```python
from build123d import *

# Parameters (mm, degrees)
EXTRUDE1_DEPTH     = 50.8
CUT_EXTRUDE1_DEPTH = 9.525
SKETCH3_R          = 2.38125
CUT_EXTRUDE2_DEPTH = 15.875
CUT_EXTRUDE3_START = -15.875
SKETCH4_R          = 2.38125
CUT_EXTRUDE3_DEPTH = 15.875
CUT_EXTRUDE4_DEPTH = 222.795964766
EXTRUDE2_DEPTH     = 50.8


with BuildPart() as part:
    # Sketch1 → Extrude1 (new body)
    with BuildSketch(Plane.XY):
        Polygon((0, 0), (215.526146874, 0), (202.826146874, 12.7), (5.260512242, 12.7), align=None)
    extrude(amount=EXTRUDE1_DEPTH)

    # Sketch2 → Cut-Extrude1 (cut)
    with BuildSketch(Plane(origin=(0, 12.7, 0), x_dir=(-1, 0, 0), z_dir=(0, 1, 0))):
        with BuildLine():
            Line((-183.776146874, 41.275), (-116.743329558, 41.275))
            ThreePointArc((-116.743329558, 41.275), (-112.253201498, 39.415128061), (-110.393329558, 34.925))
            Line((-110.393329558, 34.925), (-110.393329558, 15.875))
            ThreePointArc((-110.393329558, 15.875), (-112.253201498, 11.384871939), (-116.743329558, 9.525))
            Line((-116.743329558, 9.525), (-183.776146874, 9.525))
            ThreePointArc((-183.776146874, 9.525), (-188.266274935, 11.384871939), (-190.126146874, 15.875))
            Line((-190.126146874, 15.875), (-190.126146874, 34.925))
            ThreePointArc((-190.126146874, 34.925), (-188.266274935, 39.415128061), (-183.776146874, 41.275))
        make_face()
        with BuildLine():
            Line((-91.343329558, 9.525), (-24.310512242, 9.525))
            ThreePointArc((-24.310512242, 9.525), (-19.820384182, 11.384871939), (-17.960512242, 15.875))
            Line((-17.960512242, 15.875), (-17.960512242, 34.925))
            ThreePointArc((-17.960512242, 34.925), (-19.820384182, 39.415128061), (-24.310512242, 41.275))
            Line((-24.310512242, 41.275), (-91.343329558, 41.275))
            ThreePointArc((-91.343329558, 41.275), (-95.833457619, 39.415128061), (-97.693329558, 34.925))
            Line((-97.693329558, 34.925), (-97.693329558, 15.875))
            ThreePointArc((-97.693329558, 15.875), (-95.833457619, 11.384871939), (-91.343329558, 9.525))
        make_face()
    extrude(amount=-CUT_EXTRUDE1_DEPTH, mode=Mode.SUBTRACT)

    # Sketch3 → Cut-Extrude2 (cut)
    with BuildSketch(Plane.XY.offset(50.8)):
        with Locations((101.226146874, 6.35)):
            Circle(SKETCH3_R)
    extrude(amount=-CUT_EXTRUDE2_DEPTH, mode=Mode.SUBTRACT)

    # Sketch4 → Cut-Extrude3 (cut)
    with BuildSketch(Plane(origin=(0, 0, 0), x_dir=(-1, 0, 0), z_dir=(0, 0, -1)).offset(CUT_EXTRUDE3_START)):
        with Locations(Location((-101.226146874, 6.35, 0), (0, 0, 180))):
            Circle(SKETCH4_R)
    extrude(amount=CUT_EXTRUDE3_DEPTH, mode=Mode.SUBTRACT)

    # Sketch5 → Cut-Extrude4 (cut, through all)
    with BuildSketch(Plane.XY.offset(50.8)):
        with BuildLine():
            Line((0.800865302, 1.933459874), (0, 0))
            Line((0, 0), (10.521024484, 0))
            ThreePointArc((10.521024484, 0), (5.565730305, 0.488053878), (0.800865302, 1.933459874))
        make_face()
    extrude(amount=-CUT_EXTRUDE4_DEPTH, mode=Mode.SUBTRACT)

    # Sketch6 → Extrude2 (add)
    with BuildSketch(Plane.XY.offset(50.8)):
        with BuildLine():
            Line((5.660944893, 13.666729937), (5.260512242, 12.7))
            Line((5.260512242, 12.7), (10.521024484, 12.7))
            ThreePointArc((10.521024484, 12.7), (8.043377395, 12.944026939), (5.660944893, 13.666729937))
        make_face()
    extrude(amount=-EXTRUDE2_DEPTH)


solid = part.part
```
Verification items for the finished model (mm, model axes). A direction names the side the tool comes from. Coordinates: 2 decimals unless noted, no trailing zeros. Loops run counter-clockwise (first coordinate to the right, second up) from the corner with the lowest first, then second, coordinate; pieces in that order, holes last. Notation, with made-up numbers: (50, 20.25) - (65, 20.25) arc R23 ccw to (65, 45.25) - close; hole circle Ø3 at (29.5, 84). An arc over 180 degrees is marked (long way). Put each result on its own line as item: value.
Item 1: Set-up check for faces 4 (the face through (101, 6, 15.875)), 5 (the face through (188.22, 8, 11.34)), 6 (the face through (101, 6, 34.925)): record each of +Z, -Z, +X, -X, +Y, -Y from which the full face is reachable in a straight line by a thin tool's end or side.
Conclusion:
face 4: -Z
face 5: +Y
face 6: +Z
Item 2: Section check C-C (x = 63). Enter the section's corners in (y, z) (3 decimals).
Conclusion:
outline: (0, 0) - (12.7, 0) - (12.7, 9.525) - (3.175, 9.525) - (3.175, 41.275) - (12.7, 41.275) - (12.7, 50.8) - (0, 50.8) - close
Item 3: Gauge pin test, flat ends, axial feed: pin 1 Ø3 at (y, z) = (9.5, 25.5) entering from -X; pin 2 Ø1.4 at (x, y) = (100.5, 5.5) entering from -Z (3 decimals); pin 3 Ø7.5 at (y, z) = (8.5, 25) entering from -X. Record the tip position at first contact, or that the pin passes through.
Conclusion:
pin 1: stops at x = 3.31
pin 2: stops at z = 15.875
pin 3: stops at x = 1.97
Item 4: Section check D-D (z = 31). Enter the section's corners in (x, y) (3 decimals).
Conclusion:
outline: (0.801, 1.933) arc R25.4 ccw to (10.521, 0) - (215.526, 0) - (202.826, 12.7) - (190.126, 12.7) - (190.126, 3.175) - (110.393, 3.175) - (110.393, 12.7) - (97.693, 12.7) - (97.693, 3.175) - (17.961, 3.175) - (17.961, 12.7) - (10.521, 12.7) arc R12.7 cw to (5.661, 13.667) - close
Item 5: Section check B-B (y = 6.35). Enter the section's corners in (x, z) (3 decimals), then the cut area to 3 significant figures.
Conclusion:
outline: (2.63, 0) - (98.845, 0) - (98.845, 15.875) - (103.607, 15.875) - (103.607, 0) - (209.176, 0) - (209.176, 50.8) - (103.607, 50.8) - (103.607, 34.925) - (98.845, 34.925) - (98.845, 50.8) - (2.63, 50.8) - close; hole (17.961, 15.875) arc R6.35 ccw to (24.311, 9.525) - (91.343, 9.525) arc R6.35 ccw to (97.693, 15.875) - (97.693, 34.925) arc R6.35 ccw to (91.343, 41.275) - (24.311, 41.275) arc R6.35 ccw to (17.961, 34.925) - close; hole (110.393, 15.875) arc R6.35 ccw to (116.743, 9.525) - (183.776, 9.525) arc R6.35 ccw to (190.126, 15.875) - (190.126, 34.925) arc R6.35 ccw to (183.776, 41.275) - (116.743, 41.275) arc R6.35 ccw to (110.393, 34.925) - close
area: 5,350 mm2
Item 6: Section check A-A (z = 5.5). Enter the section's corners in (x, y), then the cut area to 3 significant figures.
Conclusion:
outline: (0.8, 1.93) arc R25.4 ccw to (10.52, 0) - (215.53, 0) - (202.83, 12.7) - (10.52, 12.7) arc R12.7 cw to (5.66, 13.67) - close; hole circle Ø4.76 at (101.23, 6.35)
area: 2,600 mm2
Item 7: Scan lines: line 1 along Z through (x, y) = (141, 5.75) (3 decimals); line 2 along X through (y, z) = (7, 14); line 3 along X through (y, z) = (4, 16). Record each from-to range of solid material in increasing order.
Conclusion:
line 1: z = 0 to 9.525, 41.275 to 50.8
line 2: x = 2.9 to 18.24, 97.41 to 98.94, 103.52 to 110.68, 189.84 to 208.53
line 3: x = 1.66 to 17.96, 97.69 to 110.39, 190.13 to 211.53
Item 8: Draft check along X on faces 1 (the face through (108, 12.7, 25)), 2 (the face through (209.265, 6.261, 25.044)), 3 (the face through (95.88, 8, 11.43)). Enter one of: pulls with the +X half, pulls with the -X half, needs draft (parallel to the pull), parting line crosses it, or undercut.
Conclusion:
face 1: needs draft
face 2: pulls with the +X half
face 3: undercut
